```python
from build123d import *

# Parameters (mm, degrees)
SKETCH_1_W               = 114
SKETCH_1_H               = 110
EXTRUDE_2_DEPTH          = 2.5
SKETCH_2_R               = 4
CUT_EXTRUDE_1_DEPTH      = 80.366239674
MIRROR_2_COPY_1_SKETCH_R = 4
MIRROR_2_COPY_1_DEPTH    = 80.366239674
HOLE_WIZARD_M3_1_D       = 2.5


with BuildPart() as part:
    # 草图1 → 凸台-拉伸2 (new, symmetric)
    with BuildSketch(Plane.XY):
        Rectangle(SKETCH_1_W, SKETCH_1_H)
    extrude(amount=EXTRUDE_2_DEPTH, both=True)

    # 草图2 → 切除-拉伸1 (cut, through all)
    with BuildSketch(Plane.XY.offset(2.5)):
        with Locations((-48, 47.5)):
            Circle(SKETCH_2_R)
    cut_extrude_1 = extrude(amount=-CUT_EXTRUDE_1_DEPTH, mode=Mode.SUBTRACT)

    # 镜向1: 切除-拉伸1 across plane
    add(cut_extrude_1.mirror(Plane.ZX), mode=Mode.SUBTRACT)

    # 镜向2: 切除-拉伸1 across plane
    add(cut_extrude_1.mirror(Plane(origin=(0, 0, 0), x_dir=(0, 0, 1), z_dir=(1, 0, 0))), mode=Mode.SUBTRACT)

    # 镜向2 copy 1 sketch → 镜向2 copy 1 (cut, through all)
    with BuildSketch(Plane(origin=(0, 0, 2.5), x_dir=(-1, 0, 0), z_dir=(0, 0, 1))):
        with Locations((-48, 47.5)):
            Circle(MIRROR_2_COPY_1_SKETCH_R)
    extrude(amount=-MIRROR_2_COPY_1_DEPTH, mode=Mode.SUBTRACT)

    # M3 螺纹孔的螺纹孔钻头1 (through all)
    with Locations(Plane(origin=(5, 15, 2.5), x_dir=(1, 0, 0), z_dir=(0, 0, 1))):
        with Locations((0, 0), (15, 0)):
            hole_wizard_m3_1 = Hole(HOLE_WIZARD_M3_1_D / 2)

    # 镜向3: M3 螺纹孔的螺纹孔钻头1 across plane
    add(hole_wizard_m3_1.mirror(Plane.ZX), mode=Mode.SUBTRACT)


solid = part.part
```
Input: part model. Units: mm. Frame: model coordinates. Round coordinates to 2 decimals unless told otherwise and drop trailing zeros. Loops run counter-clockwise (first coordinate to the right, second up) from the corner with the lowest first, then second, coordinate; pieces in that order, holes last. Notation, with made-up numbers: M 78.5,-16 L 107.5,-16 A29 ccw 107.5,9 Z; hole C 9,39 d8. An arc over 180 degrees is marked long. Answer in a Markdown table with one row per item. Add a question column.
1. Mould query, pull axis X, two halves, no side actions, for faces 1 (the face through (-1, -55, 0)), 2 (the face through (-51.2, 45.1, 0)), 3 (the face through (57, -1, 0)). Classes: released by +X, released by -X, zero draft, split by the parting line, or undercut.
2. Contact query for a flat-ended pin moving along its axis: pin 1 (5 mm diameter, centred on x = -48, y = 47.5, fed in from -Z). Output: stop coordinate, or through.
3. Ray query, probe 1 along Y at (x, z) = (5, 1.15); probe 2 along X at (y, z) = (-47.5, 0); probe 3 along Y at (x, z) = (48, 0.6). Return the intervals inside material, ascending.
4. Section C-C (z = 0.45). Give the number of separate pieces and of enclosed holes in the cut face, and give its area (3 significant figures).
5. Section B-B (x = 48). Output: boundary loops of the cut face in (y, z), and give its area (3 significant figures).
6. Section A-A (y = -47.5). Output: boundary loops of the cut face in (x, z).
Values follow:
| question | item | result |
|---|---|---|
| 1 | face 1 | zero draft |
| 1 | face 2 | undercut |
| 1 | face 3 | released by +X |
| 2 | pin 1 | through |
| 3 | probe 1 | -55 to -16.25, -13.75 to 13.75, 16.25 to 55 |
| 3 | probe 2 | -57 to -52, -44 to 44, 52 to 57 |
| 3 | probe 3 | -55 to -51.5, -43.5 to 43.5, 51.5 to 55 |
| 4 | separate pieces | 1 |
| 4 | enclosed holes | 8 |
| 4 | area | 12,300 mm^2 |
| 5 | outline | M -55,-2.5 L -51.5,-2.5 L -51.5,2.5 L -55,2.5 Z; M -43.5,-2.5 L 43.5,-2.5 L 43.5,2.5 L -43.5,2.5 Z; M 51.5,-2.5 L 55,-2.5 L 55,2.5 L 51.5,2.5 Z |
| 5 | area | 470 mm^2 |
| 6 | outline | M -57,-2.5 L -52,-2.5 L -52,2.5 L -57,2.5 Z; M -44,-2.5 L 44,-2.5 L 44,2.5 L -44,2.5 Z; M 52,-2.5 L 57,-2.5 L 57,2.5 L 52,2.5 Z |
